Geometry check sheet. Reference: the model listing, model coordinates, mm. Face numbers are marked on the shaded views. A direction names the side the tool comes from. Round coordinates to 2 decimals unless told otherwise and drop trailing zeros. Write each loop counter-clockwise with the first axis right and the second up, starting at its lowest first coordinate (ties: lowest second). Pieces come first, ordered by that corner, then holes. Notation, with made-up numbers: (65, -36) -> (79, -36) arc R19 cw to (79, -20) -> close; hole circle Ø2 at (-28, 78.5). An arc over 180 degrees is marked (long way). Use a Markdown table: item, result.
```python
from build123d import *

# Parameters (mm, degrees)
BOSS_EXTRU_1_DEPTH                  = 9
ESQUISSE2_W                         = 15.557161579
ESQUISSE2_H                         = 11.468773674
ESQUISSE2_R                         = 3
ENL_V_MAT_EXTRU_1_DEPTH             = 3
DIAM_TRE_DU_PER_AGE_2_0_2_1_D       = 2
DIAM_TRE_DU_PER_AGE_2_0_2_1_DEPTH   = 7.5
DIAM_TRE_DU_PER_AGE_2_0_2_1_TIP     = 0.600860619
DIAM_TRE_DU_PER_AGE_1_5_1_5_1_D     = 1.5
DIAM_TRE_DU_PER_AGE_1_5_1_5_1_DEPTH = 8.2
DIAM_TRE_DU_PER_AGE_1_5_1_5_1_TIP   = 0.450645464
DIAM_TRE_DU_PER_AGE_0_4_0_4_1_D     = 0.4
DIAM_TRE_DU_PER_AGE_0_4_0_4_1_DEPTH = 0.7
DIAM_TRE_DU_PER_AGE_0_4_0_4_1_TIP   = 0.120172124
ENL_V_START                         = -4
ESQUISSE3_W                         = 15.323034965
ESQUISSE3_H                         = 11.861185192
ESQUISSE3_R                         = 3
ENL_V_MAT_EXTRU_3_DEPTH             = 4
CHANFREIN2_SIZE                     = 4
CHANFREIN2_SIZE_2                   = 2.499477408


with BuildPart() as part:
    # Esquisse1 → Boss.-Extru.1 (new body)
    with BuildSketch(Plane.XY):
        Polygon((4.041451884, 0), (2.020725942, 3.5), (-2.020725942, 3.5), (-4.041451884, 0), (-2.020725942, -3.5), (2.020725942, -3.5), align=None)
    extrude(amount=BOSS_EXTRU_1_DEPTH)

    # Esquisse2 → Enlèv. mat.-Extru.1 (cut)
    with BuildSketch(Plane.XY.offset(9)):
        with Locations((-0.212602531, -0.232116366)):
            Rectangle(ESQUISSE2_W, ESQUISSE2_H)
        Circle(ESQUISSE2_R, mode=Mode.SUBTRACT)
    extrude(amount=-ENL_V_MAT_EXTRU_1_DEPTH, mode=Mode.SUBTRACT)

    # Diamètre du perçage Ø2.0 (2)1
    with Locations(Plane.XY.offset(9)):
        with Locations((0, 0)):
            Hole(DIAM_TRE_DU_PER_AGE_2_0_2_1_D / 2, depth=DIAM_TRE_DU_PER_AGE_2_0_2_1_DEPTH)
            with Locations((0, 0, -(DIAM_TRE_DU_PER_AGE_2_0_2_1_DEPTH + DIAM_TRE_DU_PER_AGE_2_0_2_1_TIP / 2))):  # 118° drill point
                Cone(0, DIAM_TRE_DU_PER_AGE_2_0_2_1_D / 2, DIAM_TRE_DU_PER_AGE_2_0_2_1_TIP, mode=Mode.SUBTRACT)

    # Diamètre du perçage Ø1.5 (1.5)1
    with Locations(Plane.XY.offset(9)):
        with Locations((0, 0)):
            Hole(DIAM_TRE_DU_PER_AGE_1_5_1_5_1_D / 2, depth=DIAM_TRE_DU_PER_AGE_1_5_1_5_1_DEPTH)
            with Locations((0, 0, -(DIAM_TRE_DU_PER_AGE_1_5_1_5_1_DEPTH + DIAM_TRE_DU_PER_AGE_1_5_1_5_1_TIP / 2))):  # 118° drill point
                Cone(0, DIAM_TRE_DU_PER_AGE_1_5_1_5_1_D / 2, DIAM_TRE_DU_PER_AGE_1_5_1_5_1_TIP, mode=Mode.SUBTRACT)

    # Diamètre du perçage Ø0.4 (0.4)1
    with Locations(Plane(origin=(0, 0, 0), x_dir=(-1, 0, 0), z_dir=(0, 0, -1))):
        with Locations((0, 0)):
            Hole(DIAM_TRE_DU_PER_AGE_0_4_0_4_1_D / 2, depth=DIAM_TRE_DU_PER_AGE_0_4_0_4_1_DEPTH)
            with Locations((0, 0, -(DIAM_TRE_DU_PER_AGE_0_4_0_4_1_DEPTH + DIAM_TRE_DU_PER_AGE_0_4_0_4_1_TIP / 2))):  # 118° drill point
                Cone(0, DIAM_TRE_DU_PER_AGE_0_4_0_4_1_D / 2, DIAM_TRE_DU_PER_AGE_0_4_0_4_1_TIP, mode=Mode.SUBTRACT)

    # Esquisse3 → Enlèv. mat.-Extru.3 (cut)
    with BuildSketch(Plane(origin=(0, 0, 0), x_dir=(-1, 0, 0), z_dir=(0, 0, -1)).offset(ENL_V_START)):
        with Locations((0.20407301, -0.146192801)):
            Rectangle(ESQUISSE3_W, ESQUISSE3_H)
        with Locations(Location((0, 0, 0), (0, 0, 180))):
            Circle(ESQUISSE3_R, mode=Mode.SUBTRACT)
    extrude(amount=ENL_V_MAT_EXTRU_3_DEPTH, mode=Mode.SUBTRACT)

    # Chanfrein2
    # the kernel refuses this chamfer: 4, 2.499477408 mm, written as the material it takes off along each edge
    with BuildSketch(Plane(origin=(0, 0, 0), x_dir=(1, 0, 0), z_dir=(0, 1, 0))) as chanfrein2_piece_1_section:
        Polygon((3, -CHANFREIN2_SIZE), (3 - CHANFREIN2_SIZE_2, 0), (3, 0), align=None)
    chanfrein2_piece_1 = revolve(axis=Axis((0, 0, 0), (0, 0, -1)), mode=Mode.PRIVATE)
    chanfrein2_piece_1 = split(chanfrein2_piece_1, bisect_by=Plane(origin=(-1.744026904, 0, 4), z_dir=(0, 0, -1)), keep=Keep.TOP, mode=Mode.PRIVATE)
    add(chanfrein2_piece_1, mode=Mode.SUBTRACT)


solid = part.part
```
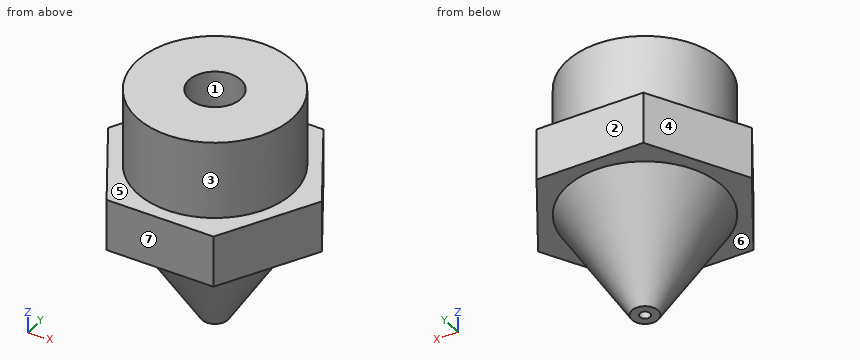
(1) Release check for a two-part mould opening along X. For the marked faces 1, 2, 3 and 4 record: +X half, -X half, draft (parallel to the pull), parting line (faces both ways), or undercut.
A:
| item | result |
|---|---|
| face 1 | undercut |
| face 2 | draft |
| face 3 | parting line |
| face 4 | -X half |
(2) Thickness scan on line 1 (Y direction, x = 0, z = 8); line 2 (Z direction, x = 1.75, y = -2.75); line 3 (X direction, y = -0.5, z = 2.75). Record the ranges inside material, lowest first.
A:
| item | result |
|---|---|
| line 1 | y = -3 to -1, 1 to 3 |
| line 2 | z = 4 to 6 |
| line 3 | x = -2.16 to -0.87, 0.87 to 2.16 |
(3) Gauge pin test, flat ends, axial feed: pin 1 Ø1.2 at (x, y) = (0, 0) entering from +Z; pin 2 Ø1.7 at (x, y) = (0, 0) entering from +Z; pin 3 Ø3 at (x, y) = (-3, 2) entering from -Z. Record the tip position at first contact, or that the pin passes through.
A:
| item | result |
|---|---|
| pin 1 | stops at z = 0.71 |
| pin 2 | stops at z = 1.41 |
| pin 3 | stops at z = 2.57 |
(4) Access from +Z, -Z, +X, -X, +Y, -Y to the whole of each face (thin tool, end or side, straight path). Record for the marked faces 5, 6 and 7.
A:
| item | result |
|---|---|
| face 5 | +Z |
| face 6 | -Z |
| face 7 | +Z, -Z, +X, -X, -Y |
(5) Section check A-A on x = 0. Record the cut outline in (y, z).
A:
| item | result |
|---|---|
| outline | (-3.5, 4) -> (-3, 4) -> (-0.5, 0) -> (-0.2, 0) -> (-0.2, 0.47) -> (-0.75, 0.8) -> (-0.75, 1.35) -> (-1, 1.5) -> (-1, 9) -> (-3, 9) -> (-3, 6) -> (-3.5, 6) -> close; (0.2, 0) -> (0.5, 0) -> (3, 4) -> (3.5, 4) -> (3.5, 6) -> (3, 6) -> (3, 9) -> (1, 9) -> (1, 1.5) -> (0.75, 1.35) -> (0.75, 0.8) -> (0.2, 0.47) -> close |
(6) Section check B-B on x = -3.25. Record the cut outline in (y, z).
A:
| item | result |
|---|---|
| outline | (-1.37, 4) -> (1.37, 4) -> (1.37, 6) -> (-1.37, 6) -> close |
